Read the model definition and answer for the solid it produces. Units are mm, in the model's axes. A direction names the side the tool comes from. Give positions to 0.01 mm unless a question says otherwise; leave off trailing zeros. Order: outer loops, then holes, each group sorted by start corner. A loop starts at its lowest first (then second) coordinate and runs counter-clockwise, first axis right, second up. Notation, with made-up numbers: M 72.5,82 L 126.5,82 A30 ccw 126.5,117 Z; hole C -18,-1 d9. An arc over 180 degrees is marked long. One line per item, written item: value.
Autodesk Inventor part; units mm, degrees
ref_plane "YZ Plane" through (0, 0, 0) normal (1, 0, 0) x (0, 1, 0)
ref_plane "XZ Plane" through (0, 0, 0) normal (0, 1, 0) x (-1, 0, 0)
ref_plane "XY Plane" through (0, 0, 0) normal (0, 0, 1) x (1, 0, 0)
sketch "Sketch1" plane through (0, 0, 0) normal (0, 0, 1) x (1, 0, 0)
  circle A0 centre (0, 0) radius 8
  dimension "d0" = 16
extrude "Extrusion1" add sketch "Sketch1" along normal blind 82
sketch "Sketch2" plane through (0, 0, 82) normal (0, 0, 1) x (1, 0, 0)
  circle A0 centre (0, 0) radius 6
  dimension "d4" = 12
extrude "Extrusion2" add sketch "Sketch2" along normal blind 11
sketch "Sketch3" plane through (0, 0, 93) normal (0, 0, 1) x (1, 0, 0)
  circle A0 centre (0, 0) radius 4
  dimension "d7" = 8
extrude "Extrusion3" add sketch "Sketch3" along normal blind 5
sketch "Sketch4" plane through (0, 0, 98) normal (0, 0, 1) x (1, 0, 0)
  circle A0 centre (0, 0) radius 6
  dimension "d10" = 12
extrude "Extrusion4" add sketch "Sketch4" along normal blind 6
sketch "Sketch5" plane through (0, 0, 0) normal (0, 0, -1) x (-1, 0, 0)
  circle A0 centre (0, 0) radius 6
  dimension "d13" = 12
extrude "Extrusion5" add sketch "Sketch5" along normal blind 10
sketch "Sketch6" plane through (0, 0, -10) normal (0, 0, -1) x (-1, 0, 0)
  circle A0 centre (0, 0) radius 9
  dimension "d16" = 18
extrude "Extrusion6" add sketch "Sketch6" along normal blind 24
sketch "Sketch7" plane through (0, 0, 0) normal (1, 0, 0) x (0, 1, 0)
  line L0 (-9, -10) -> (9, -10)
  line L1 (-9, -34) -> (9, -34)
  line L2 (-9, -10) -> (9, -34)
  line L3 (9, -10) -> (-9, -34)
  circle A0 centre (0, -22) radius 3
  point P0 (0, 0)
  dimension "d19" = 6
extrude "Extrusion7" cut sketch "Sketch7" against normal mid plane 24 contours A0 L3 L2 | L2 L3 A0 | A0 L2 L3 | L2 A0 L3
properties part number "09.TornilloSinFin.LPSM" material "Steel, Alloy"
1) Find section C-C, the plane z = -22. Write down the section's boundary in (x, y), plus the area to 3 significant figures.
Reported:
outline: M -8.49,-3 A9 ccw 8.49,-3 Z; M -8.49,3 L 8.49,3 A9 ccw Z
area: 149 mm^2
2) Each of these flat-tipped pins is pushed along its axis until it touches: pin 1 Ø1 at (y, z) = (-4.5, 80) entering from -X; pin 2 Ø5 at (x, z) = (-1, 64) entering from -Y; pin 3 Ø8 at (y, z) = (0, 13.5) entering from +X. Where does it stop, or does it pass through?
Reported:
pin 1: stops at x = -6.93
pin 2: stops at y = -8
pin 3: stops at x = 8
3) Which of the six approach directions +Z, -Z, +X, -X, +Y, -Y give full straight-line access (tool end or side, diameter ignored) to faces 1 (the face through (-6, 0, 101)), 2 (the face through (-1.42, -3.92, 93)), 3 (the face through (0, 0, -34))?
Reported:
face 1: +Z
face 2: none
face 3: -Z, +X, -X, +Y, -Y
4) Consider probe 1 along Z at (x, y) = (-3.25, -6.75); probe 2 along Z at (x, y) = (2.5, 0); probe 3 along Y at (x, z) = (0.25, 73.5). Determine where each line is inside the solid, lowest interval first.
Reported:
probe 1: z = -34 to -10, 0 to 82
probe 2: z = -34 to -25, -19 to 104
probe 3: y = -8 to 8
5) Find section B-B, the plane y = 0. Write down the section's boundary in (x, z).
Reported:
outline: M -9,-34 L 9,-34 L 9,-25 L -9,-25 Z; M -9,-19 L 9,-19 L 9,-10 L 6,-10 L 6,0 L 8,0 L 8,82 L 6,82 L 6,93 L 4,93 L 4,98 L 6,98 L 6,104 L -6,104 L -6,98 L -4,98 L -4,93 L -6,93 L -6,82 L -8,82 L -8,0 L -6,0 L -6,-10 L -9,-10 Z
6) Determine the mould class of faces 4 (the face through (-1.73, 7.81, 40.43)), 5 (the face through (-2, -6, -10)), 6 (the face through (-2, 6, 82)) for opening direction Z: +Z half, -Z half, draft (parallel to the pull), parting line (faces both ways), or undercut.
Reported:
face 4: draft
face 5: undercut
face 6: +Z half
7) Find section D-D, the plane z = 60. Write down the section's boundary in (x, y).
Reported:
outline: C 0,0 d16
8) Find section A-A, the plane x = 0. Write down the section's boundary in (y, z), plus the area to 3 significant figures.
Reported:
outline: M -9,-34 L 9,-34 L 9,-10 L 6,-10 L 6,0 L 8,0 L 8,82 L 6,82 L 6,93 L 4,93 L 4,98 L 6,98 L 6,104 L -6,104 L -6,98 L -4,98 L -4,93 L -6,93 L -6,82 L -8,82 L -8,0 L -6,0 L -6,-10 L -9,-10 Z; hole C 0,-22 d6
area: 2,080 mm^2
